from build123d import *

# Parameters (mm, degrees)
SKETCH1_R           = 7.5
BOSS_EXTRUDE1_DEPTH = 24
SKETCH2_R           = 4
CUT_EXTRUDE1_DEPTH  = 24
FILLET2_R           = 0.3
FILLET3_R           = 0.3
SKETCH3_R           = 7.2
SKETCH3_R_2         = 4.3
CUT_EXTRUDE2_DEPTH  = 0.3
CUT_EXTRUDE4_START  = -0.3
SKETCH4_R           = 7.2
SKETCH4_R_2         = 4.3
CUT_EXTRUDE4_DEPTH  = 0.3


with BuildPart() as part:
    # Sketch1 → Boss-Extrude1 (new body)
    with BuildSketch(Plane.XY):
        Circle(SKETCH1_R)
    extrude(amount=BOSS_EXTRUDE1_DEPTH)

    # Sketch2 → Cut-Extrude1 (cut)
    with BuildSketch(Plane.XY.offset(24)):
        Circle(SKETCH2_R)
    extrude(amount=-CUT_EXTRUDE1_DEPTH, mode=Mode.SUBTRACT)

    # Fillet2
    fillet2_edges = [part.edges().sort_by_distance(p)[0] for p in [
        (-4, 0, 0),
        (-4, 0, 24),
    ]]
    fillet(fillet2_edges, radius=FILLET2_R)

    # Fillet3
    fillet3_edges = [part.edges().sort_by_distance(p)[0] for p in [
        (-7.5, 0, 0),
        (-7.5, 0, 24),
    ]]
    fillet(fillet3_edges, radius=FILLET3_R)

    # Sketch3 → Cut-Extrude2 (cut)
    with BuildSketch(Plane(origin=(0, 0, 0), x_dir=(-1, 0, 0), z_dir=(0, 0, -1))):
        Circle(SKETCH3_R)
        Circle(SKETCH3_R_2, mode=Mode.SUBTRACT)
    extrude(amount=-CUT_EXTRUDE2_DEPTH, mode=Mode.SUBTRACT)

    # Sketch4 → Cut-Extrude4 (cut)
    with BuildSketch(Plane.XY.offset(24).offset(CUT_EXTRUDE4_START)):
        with Locations(Location((0, 0, 0), (0, 0, 180))):
            Circle(SKETCH4_R)
        with Locations(Location((0, 0, 0), (0, 0, 180))):
            Circle(SKETCH4_R_2, mode=Mode.SUBTRACT)
    extrude(amount=CUT_EXTRUDE4_DEPTH, mode=Mode.SUBTRACT)


solid = part.part
Verification items for the finished model (mm, model axes). A direction names the side the tool comes from. Round coordinates to 2 decimals unless told otherwise and drop trailing zeros. Order: outer loops, then holes, each group sorted by start corner. A loop starts at its lowest first (then second) coordinate and runs counter-clockwise, first axis right, second up.
1. Section check C-C on z = 9.75. Record the cut outline in (x, y).
Final values:
outline: circle Ø15 at (0, 0); hole circle Ø8 at (0, 0)
2. Release check for a two-part mould opening along X. For faces 4 (the cylindrical face through (3.41, 2.62, 23.85)), 5 (the cylindrical face through (-7.493, 0.33, 11.836)) record: +X half, -X half, draft (parallel to the pull), parting line (faces both ways), or undercut.
Final values:
face 4: undercut
face 5: parting line
3. Access from +Z, -Z, +X, -X, +Y, -Y to the whole of each face (thin tool, end or side, straight path). Record for faces 1 (the cylindrical face through (-0.867, -3.905, 12.164)), 2 (the flat face through (0, -5, 0.3)), 3 (the flat face through (0, 5, 23.7)).
Final values:
face 1: +Z, -Z
face 2: -Z
face 3: +Z
4. Thickness scan on L1, parallel to Y at x = 0, z = 9; L2, parallel to Y at x = 1.5, z = 17.5; L3, parallel to Z at x = -2.25, y = -6. Record the ranges inside material, lowest first.
Final values:
L1: y = -7.5 to -4, 4 to 7.5
L2: y = -7.35 to -3.71, 3.71 to 7.35
L3: z = 0.3 to 23.7
5. Section check A-A on y = 0. Record the cut outline in (x, z), then the cut area to 3 significant figures.
Final values:
outline: (-7.5, 0.3) arc R0.3 ccw to (-7.2, 0) - (-7.2, 0.3) - (-4.3, 0.3) - (-4.3, 0) arc R0.3 ccw to (-4, 0.3) - (-4, 23.7) arc R0.3 ccw to (-4.3, 24) - (-4.3, 23.7) - (-7.2, 23.7) - (-7.2, 24) arc R0.3 ccw to (-7.5, 23.7) - close; (4, 0.3) arc R0.3 ccw to (4.3, 0) - (4.3, 0.3) - (7.2, 0.3) - (7.2, 0) arc R0.3 ccw to (7.5, 0.3) - (7.5, 23.7) arc R0.3 ccw to (7.2, 24) - (7.2, 23.7) - (4.3, 23.7) - (4.3, 24) arc R0.3 ccw to (4, 23.7) - close
area: 164 mm2
6. Go/stop test with flat-tipped pins: P1, Ø4, axis at x = 4.5, z = 14, coming from the -Y side; P2, Ø1, axis at y = -4, z = 17, coming from the -X side. Record where each tip stops, or that it passes through.
Final values:
P1: stops at y = -7.07
P2: stops at x = -6.63
